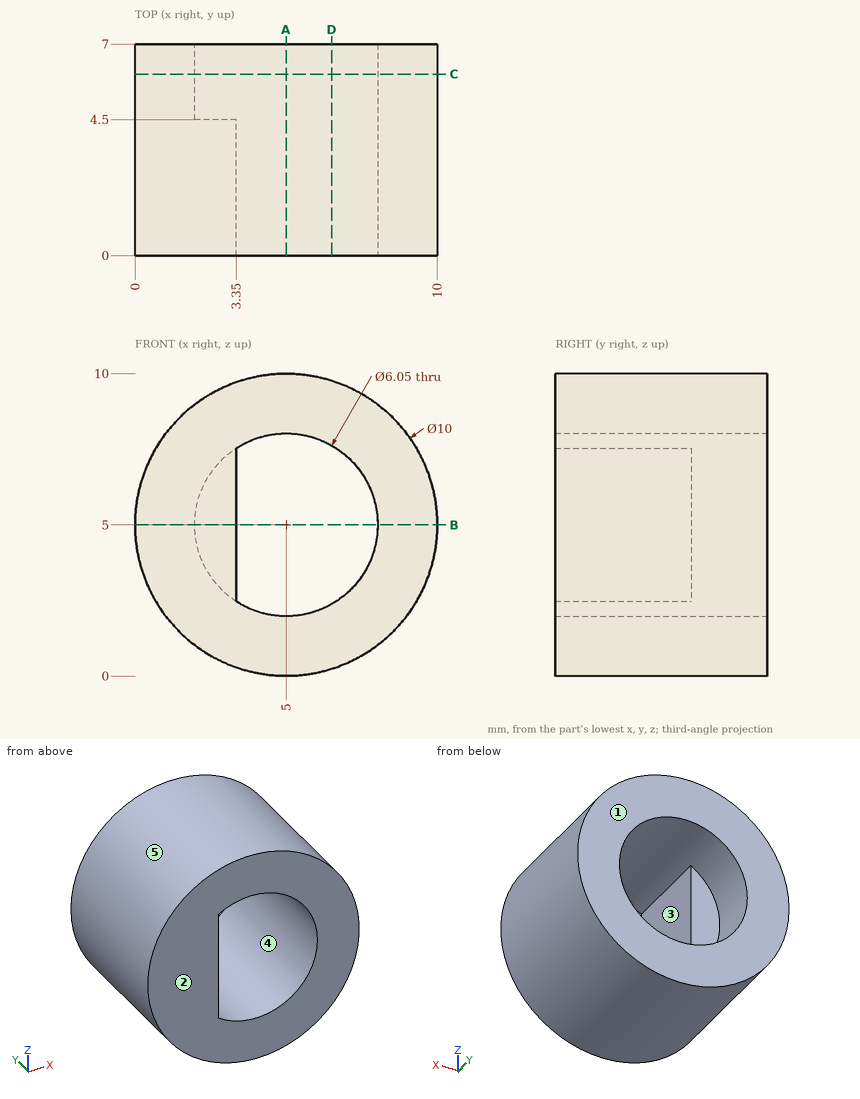
Study the drawing (mm; zero at the part's minimum x, y, z) and answer. A direction names the side the tool comes from. Give positions to 0.01 mm unless a question says otherwise; leave off trailing zeros. Write each loop counter-clockwise with the first axis right and the second up, starting at its lowest first coordinate (ties: lowest second). Pieces come first, ordered by that corner, then holes.
Item 1: Section D-D, the plane x = 6.5 is taken. Write down the section's boundary in (y, z).
Item 2: Determine the mould class of the marked faces 1, 2 and 3 for opening direction Y: released by +Y, released by -Y, zero draft, split by the parting line, or undercut.
Item 3: Section A-A, the plane x = 5 is taken. Write down the section's boundary in (y, z) (3 decimals).
Item 4: Find the intervals of material crossed by line 1 along X through (y, z) = (5.75, 5) (3 decimals); line 2 along X through (y, z) = (3.25, 5) (3 decimals), in increasing order.
Item 5: Section B-B, the plane z = 5 is taken. Write down the section's boundary in (x, y) (3 decimals), plus the area to 3 significant figures.
Item 6: Which of the six approach directions +Z, -Z, +X, -X, +Y, -Y give full straight-line access (tool end or side, diameter ignored) to the marked faces 4 and 5?
Item 7: Flat-ended cylindrical pins translate along their axes: P1, Ø4, axis at y = 1, z = 2.5, coming from the -X side; P2, Ø1.5, axis at y = 3.5, z = 8, coming from the -X side. Find the tip coordinate at first contact, or state that the pin passes through.
Item 8: Section C-C, the plane y = 6 is taken. Write down the section's boundary in (x, z) (3 decimals), plus the area to 3 significant figures.
Completed:
1. outline: (0, 0.23) - (7, 0.23) - (7, 2.37) - (0, 2.37) - close; (0, 7.63) - (7, 7.63) - (7, 9.77) - (0, 9.77) - close
2. face 1: released by +Y
2. face 2: released by -Y
2. face 3: zero draft
3. outline: (0, 0) - (7, 0) - (7, 1.975) - (0, 1.975) - close; (0, 8.025) - (7, 8.025) - (7, 10) - (0, 10) - close
4. line 1: x = 0 to 1.975, 8.025 to 10
4. line 2: x = 0 to 3.35, 8.025 to 10
5. outline: (0, 0) - (3.35, 0) - (3.35, 4.5) - (1.975, 4.5) - (1.975, 7) - (0, 7) - close; (8.025, 0) - (10, 0) - (10, 7) - (8.025, 7) - close
5. area: 33.8 mm2
6. face 4: +Y
6. face 5: +Y, -Y
7. P1: stops at x = 0.03
7. P2: stops at x = 0.53
8. outline: circle Ø10 at (5, 5); hole circle Ø6.05 at (5, 5)
8. area: 49.8 mm2
